The listing builds one solid part. Answer for the finished solid, in the listing's coordinates (mm). Coordinates: 2 decimals unless noted, no trailing zeros. Loops run counter-clockwise (first coordinate to the right, second up) from the corner with the lowest first, then second, coordinate; pieces in that order, holes last. Notation, with made-up numbers: (-28, 78) - (-13, 78) arc R20 ccw to (-13, 88) - close; hole circle Ø10 at (38.25, 47). An arc over 180 degrees is marked (long way). Put each result on its own line as item: value.
```python
from build123d import *

# Parameters (mm, degrees)
SKETCH_1_W          = 150
SKETCH_1_H          = 114
EXTRUDE_1_DEPTH     = 3
SKETCH_2_R          = 1.5
SKETCH_2_R_2        = 5
CUT_EXTRUDE_1_DEPTH = 3


with BuildPart() as part:
    # 草图1 → 凸台-拉伸1 (new body)
    with BuildSketch(Plane(origin=(0, 0, 0), x_dir=(1, 0, 0), z_dir=(0, 1, 0))):
        with Locations((75, -57)):
            Rectangle(SKETCH_1_W, SKETCH_1_H)
    extrude(amount=EXTRUDE_1_DEPTH)

    # 草图2 → 切除-拉伸1 (cut)
    with BuildSketch(Plane(origin=(0, 3, 0), x_dir=(1, 0, 0), z_dir=(0, 1, 0))):
        with Locations((25, -57)):
            Circle(SKETCH_2_R)
        with Locations((101.3, -75)):
            Circle(SKETCH_2_R)
        with Locations((101.3, -39)):
            Circle(SKETCH_2_R)
        with Locations((71.3, -80.5)):
            Circle(SKETCH_2_R)
        with Locations((46.3, -80.5)):
            Circle(SKETCH_2_R)
        with Locations((71.3, -33.5)):
            Circle(SKETCH_2_R)
        with Locations((46.3, -33.5)):
            Circle(SKETCH_2_R)
        with Locations((81.3, -57)):
            Circle(SKETCH_2_R_2)
    extrude(amount=-CUT_EXTRUDE_1_DEPTH, mode=Mode.SUBTRACT)


solid = part.part
```
1) The part is cut by section A-A (x = 81.3). Give the vertices of the cut face in (y, z), and give its area (3 significant figures).
Found:
outline: (0, 0) - (3, 0) - (3, 52) - (0, 52) - close; (0, 62) - (3, 62) - (3, 114) - (0, 114) - close
area: 312 mm^2
2) For a pull along Z with two mould halves and no side action, classify faces 1 (the face through (101.99, 1.52, 40.33)), 2 (the face through (74, 0, 56)), 3 (the face through (74, 1, 0)) as pulls with the +Z half, pulls with the -Z half, needs draft (parallel to the pull), parting line crosses it, or undercut.
Found:
face 1: undercut
face 2: needs draft
face 3: pulls with the -Z half
3) Straight lines are drawn through the part: L1, parallel to X at y = 1.7, z = 80.5; L2, parallel to Z at x = 101.3, y = 2.1; L3, parallel to Z at x = 25, y = 1.35. For each, find the intervals that lie inside material, in ascending order. Write a range as [from, to].
Found:
L1: x = [0, 44.8], [47.8, 69.8], [72.8, 150]
L2: z = [0, 37.5], [40.5, 73.5], [76.5, 114]
L3: z = [0, 55.5], [58.5, 114]
